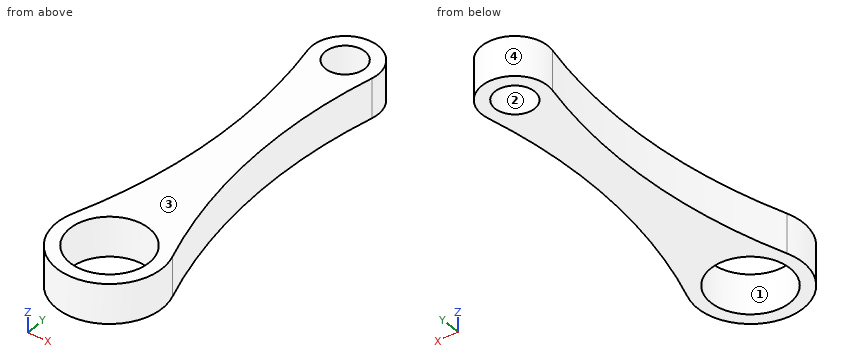
Autodesk Inventor part; units mm, degrees
ref_plane "YZ Plane" through (0, 0, 0) normal (1, 0, 0) x (0, 1, 0)
ref_plane "XZ Plane" through (0, 0, 0) normal (0, 1, 0) x (-1, 0, 0)
ref_plane "XY Plane" through (0, 0, 0) normal (0, 0, 1) x (1, 0, 0)
sketch "Sketch1" plane through (0, 0, 0) normal (0, 0, 1) x (1, 0, 0)
  circle A0 centre (0, 0) radius 9.525
  circle A1 centre (0, -152.4) radius 19.05
  line L0 (0, -216.535) -> (0, 54.61) construction
  circle A2 centre (0, 0) radius 15.875
  circle A3 centre (0, -152.4) radius 25.4
  arc A4 (-23.9399, -143.9123) -> (-15.4905, -3.4727) centre (-263.3389, -59.0352) ccw
  arc A5 (15.4905, -3.4727) -> (23.9399, -143.9123) centre (263.3389, -59.0352) ccw
  point P0 (23.9399, -143.9123)
  point P1 (15.4905, -3.4727)
  dimension "d0" = 19.05
  dimension "d1" = 38.1
  dimension "conrod_ctc" = 152.4
  dimension "conrod_wt" = 6.35
  dimension "d5" = 6.35
  dimension "conrod_rad" = 254
extrude "Extrusion1" add sketch "Sketch1" along normal mid plane 19.05
equation "\"d0\" = pin_dia"
equation "\"d1\" = 2 * d0"
equation "\"d5\" = conrod_wt"
properties part number "Connecting_Rod" material "Titanium"
CAD build for the part. Positions are in the model's coordinates, mm. Face numbers are marked on the shaded views. Round coordinates to 2 decimals unless told otherwise and drop trailing zeros. Write each loop counter-clockwise with the first axis right and the second up, starting at its lowest first coordinate (ties: lowest second). Pieces come first, ordered by that corner, then holes.
(1) Probe line 1 along Y through (x, z) = (0, 0.75) (3 decimals); line 2 along Y through (x, z) = (3, 5); line 3 along X through (y, z) = (-149, -5.5). List the from-to ranges inside material, lowest first.
(2) Slice it at B-B, the plane x = 0. Write the cut outline in (y, z) (3 decimals), and give its area (3 significant figures).
(3) Slice it at A-A, the plane y = 0. Write the cut outline in (x, z) (3 decimals).
(4) Slice it at C-C, the plane z = 1.75. Count the separate pieces of the cut face and the enclosed holes in it, and give its area (3 significant figures).
(5) Drop flat-ended pins along their axis: P1, Ø5, axis at x = 3, z = 3, coming from the +Y side; P2, Ø2, axis at x = -7.5, z = -3, coming from the -Y side; P3, Ø1, axis at y = -109, z = 0, coming from the -X side; P4, Ø11.5, axis at x = 0, y = 0, coming from the +Z side. Give the stop position or say it passes through.
(6) Mould opens along X. For the marked faces 1, 2, 3 and 4 say: pulls with the +X half, pulls with the -X half, needs draft (parallel to the pull), parting line crosses it, or undercut.
(7) Slice it at D-D, the plane y = -146.5. Write the cut outline in (x, z) (3 decimals), and give its area (3 significant figures).
From the geometry:
1. line 1: y = -177.8 to -171.45, -133.35 to -9.525, 9.525 to 15.875
1. line 2: y = -177.62 to -171.21, -133.59 to -9.04, 9.04 to 15.59
1. line 3: x = -25.17 to -18.74, 18.74 to 25.17
2. outline: (-177.8, -9.525) - (-171.45, -9.525) - (-171.45, 9.525) - (-177.8, 9.525) - close; (-133.35, -9.525) - (-9.525, -9.525) - (-9.525, 9.525) - (-133.35, 9.525) - close; (9.525, -9.525) - (15.875, -9.525) - (15.875, 9.525) - (9.525, 9.525) - close
2. area: 2,600 mm2
3. outline: (-15.875, -9.525) - (-9.525, -9.525) - (-9.525, 9.525) - (-15.875, 9.525) - close; (9.525, -9.525) - (15.875, -9.525) - (15.875, 9.525) - (9.525, 9.525) - close
4. separate pieces: 1
4. enclosed holes: 2
4. area: 4,180 mm2
5. P1: stops at y = 15.87
5. P2: stops at y = -176.95
5. P3: stops at x = -14.4
5. P4: passes through
6. face 1: undercut
6. face 2: undercut
6. face 3: needs draft
6. face 4: parting line crosses it
7. outline: (-24.705, -9.525) - (-18.113, -9.525) - (-18.113, 9.525) - (-24.705, 9.525) - close; (18.113, -9.525) - (24.705, -9.525) - (24.705, 9.525) - (18.113, 9.525) - close
7. area: 251 mm2
